Check sheet for the modelled part. Datum: model origin and axes. Units: mm. Face numbers are marked on the shaded views. A direction names the side the tool comes from. Give positions to 0.01 mm unless a question says otherwise; leave off trailing zeros. Write each loop counter-clockwise with the first axis right and the second up, starting at its lowest first coordinate (ties: lowest second). Pieces come first, ordered by that corner, then holes. Notation, with made-up numbers: (25.5, -9) -> (47.5, -9) arc R18 ccw to (47.5, 12) -> close; hole circle Ø2 at (70.25, 15.5). An arc over 180 degrees is marked (long way). Answer as a JSON object with one key per item and string values.
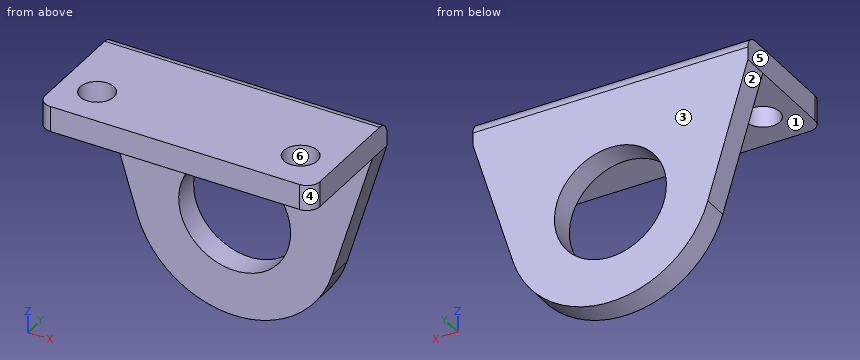
from build123d import *

# Parameters (mm, degrees)
CROQUIS1_R              = 11
SALIENTE_EXTRUIR1_DEPTH = 5
CROQUIS2_W              = 54
CROQUIS2_H              = 25
CROQUIS2_R              = 3.3
SALIENTE_EXTRUIR2_DEPTH = 5
REDONDEO1_R             = 2.5
REDONDEO2_R             = 2.5


with BuildPart() as part:
    # Croquis1 → Saliente-Extruir1 (new body)
    with BuildSketch(Plane(origin=(0, 0, 0), x_dir=(1, 0, 0), z_dir=(0, 1, 0))):
        with BuildLine():
            Line((-27, 0), (27, 0))
            Line((27, 0), (27, 5))
            Line((27, 5), (19.131975199, 30.828166519))
            ThreePointArc((19.131975199, 30.828166519), (0, 45), (-19.131975199, 30.828166519))
            Line((-19.131975199, 30.828166519), (-27, 5))
            Line((-27, 5), (-27, 0))
        make_face()
        with Locations(Location((0, 25, 0), (0, 0, 270))):
            Circle(CROQUIS1_R, mode=Mode.SUBTRACT)
    extrude(amount=-SALIENTE_EXTRUIR1_DEPTH)

    # Croquis2 → Saliente-Extruir2 (add)
    with BuildSketch(Plane.XY):
        with Locations((0, -12.5)):
            Rectangle(CROQUIS2_W, CROQUIS2_H)
        with Locations((20, -17)):
            Circle(CROQUIS2_R, mode=Mode.SUBTRACT)
        with Locations((-20, -17)):
            Circle(CROQUIS2_R, mode=Mode.SUBTRACT)
    extrude(amount=-SALIENTE_EXTRUIR2_DEPTH)

    # Redondeo1
    redondeo1_edges = [part.edges().sort_by_distance(p)[0] for p in [
        (0, 0, 0),
    ]]
    fillet(redondeo1_edges, radius=REDONDEO1_R)

    # Redondeo2
    redondeo2_edges = [part.edges().sort_by_distance(p)[0] for p in [
        (-27, -25, -2.5),
        (27, -25, -2.5),
    ]]
    fillet(redondeo2_edges, radius=REDONDEO2_R)


solid = part.part
1. Sectioned sample at D-D, the plane z = -25. Enter the section's corners in (x, y).
Determined:
{"outline": "(-20.91, -5) -> (-11, -5) -> (-11, 0) -> (-20.91, 0) -> close; (11, -5) -> (20.91, -5) -> (20.91, 0) -> (11, 0) -> close"}
2. Sectioned sample at A-A, the plane x = 0. Enter the section's corners in (y, z).
Determined:
{"outline": "(-25, -5) -> (-5, -5) -> (-5, -14) -> (0, -14) -> (0, -2.5) arc R2.5 ccw to (-2.5, 0) -> (-25, 0) -> close; (-5, -45) -> (0, -45) -> (0, -36) -> (-5, -36) -> close"}
3. Scan lines: L1, parallel to Z at x = 12, y = -19; L2, parallel to Y at x = 20, z = -1. Record each from-to range of solid material in increasing order. Write a range as [from, to].
Determined:
{"L1": "[-5, 0]", "L2": "[-25, -20.3], [-13.7, -0.5]"}
4. Sectioned sample at C-C, the plane y = -17. Enter the section's corners in (x, z).
Determined:
{"outline": "(-27, -5) -> (-23.3, -5) -> (-23.3, 0) -> (-27, 0) -> close; (-16.7, -5) -> (16.7, -5) -> (16.7, 0) -> (-16.7, 0) -> close; (23.3, -5) -> (27, -5) -> (27, 0) -> (23.3, 0) -> close"}
5. Access from +Z, -Z, +X, -X, +Y, -Y to the whole of each face (thin tool, end or side, straight path). Record for the marked faces 1 and 2.
Determined:
{"face 1": "-Z, +X, -X, -Y", "face 2": "-Z, -X, +Y, -Y"}
6. Mould release check, pull along Y, two halves, no side actions. Record for the marked faces 3, 4, 5 and 6: released by +Y, released by -Y, zero draft, split by the parting line, or undercut.
Determined:
{"face 3": "released by +Y", "face 4": "released by -Y", "face 5": "zero draft", "face 6": "undercut"}
7. Go/stop test with flat-tipped pins: P1, Ø5.5, axis at x = -20, y = -17, coming from the +Z side; P2, Ø4, axis at x = -18.5, z = -19.5, coming from the +Y side; P3, Ø12, axis at x = 11, z = -32, coming from the -Y side; P4, Ø5, axis at x = -11, y = -10, coming from the -Z side. Record where each tip stops, or that it passes through.
Determined:
{"P1": "through", "P2": "y = 0", "P3": "y = -5", "P4": "z = -5"}
8. Sectioned sample at B-B, the plane y = -4. Enter the section's corners in (x, z).
Determined:
{"outline": "(-27, -5) -> (-19.13, -30.83) arc R20 ccw to (19.13, -30.83) -> (27, -5) -> (27, 0) -> (-27, 0) -> close; hole circle Ø22 at (0, -25)"}
